Check sheet for the modelled part. Datum: model origin and axes. Units: mm. Face numbers are marked on the shaded views. Round coordinates to 2 decimals unless told otherwise and drop trailing zeros. Loops run counter-clockwise (first coordinate to the right, second up) from the corner with the lowest first, then second, coordinate; pieces in that order, holes last. Notation, with made-up numbers: (10, 39) - (43, 39) arc R12 cw to (43, 61) - close; hole circle Ø3 at (76, -39.75). An arc over 180 degrees is marked (long way). Put each result on its own line as item: value. Start each with the question number.
Item 1: Material ranges on line 1 along X through (y, z) = (1.15, 0); line 2 along X through (y, z) = (3.9, 0); line 3 along X through (y, z) = (4.8, -18), recorded low to high.
Item 2: Section check D-D, the plane z = -24.5. Record the cut outline in (x, y).
Item 3: Section check A-A, the plane y = 3.85. Record the cut outline in (x, z), and give its area (3 significant figures).
Item 4: Gauge pin test, flat ends, axial feed: pin 1 Ø0.9 at (x, z) = (-18, 18) entering from +Y; pin 2 Ø0.8 at (x, y) = (-1, 2) entering from +Z; pin 3 Ø4 at (x, z) = (33, 0) entering from -Y. Record the tip position at first contact, or that the pin passes through.
Item 5: Section check B-B, the plane z = 33.1. Record the cut outline in (x, y), and give its area (3 significant figures).
Item 6: Draft check along Z on the marked faces 1 and 2. Enter one of: pulls with the +Z half, pulls with the -Z half, needs draft (parallel to the pull), parting line crosses it, or undercut.
Item 7: Section check C-C, the plane x = -33.1. Record the cut outline in (y, z).
from build123d import *

# Parameters (mm, degrees)
SKETCH1_R           = 38.1
BOSS_EXTRUDE1_DEPTH = 5
SKETCH3_W           = 8.5
SKETCH3_H           = 20.2
CUT_EXTRUDE2_DEPTH  = 2.5
SKETCH4_W           = 5
SKETCH4_H           = 2
CUT_EXTRUDE4_DEPTH  = 54.939503149
SKETCH5_R           = 1.5
CUT_EXTRUDE5_DEPTH  = 3
SKETCH6_R           = 2.5
CUT_EXTRUDE6_DEPTH  = 3


with BuildPart() as part:
    # Sketch1 → Boss-Extrude1 (new body)
    with BuildSketch(Plane(origin=(0, 0, 0), x_dir=(1, 0, 0), z_dir=(0, 1, 0))):
        with Locations(Location((0, 0, 0), (0, 0, 270))):
            Circle(SKETCH1_R)
    extrude(amount=BOSS_EXTRUDE1_DEPTH)

    # Sketch3 → Cut-Extrude2 (cut)
    with BuildSketch(Plane(origin=(0, 5, 0), x_dir=(1, 0, 0), z_dir=(0, 1, 0))):
        with Locations((0, 7.5)):
            Rectangle(SKETCH3_W, SKETCH3_H)
    extrude(amount=-CUT_EXTRUDE2_DEPTH, mode=Mode.SUBTRACT)

    # Sketch4 → Cut-Extrude4 (cut, through all)
    with BuildSketch(Plane(origin=(0, 2.5, 0), x_dir=(1, 0, 0), z_dir=(0, 1, 0))):
        with Locations((0, -1.6)):
            Rectangle(SKETCH4_W, SKETCH4_H)
    extrude(amount=-CUT_EXTRUDE4_DEPTH, mode=Mode.SUBTRACT)

    # Sketch5 → Cut-Extrude5 (cut)
    with BuildSketch(Plane(origin=(0, 5, 0), x_dir=(1, 0, 0), z_dir=(0, 1, 0))):
        with Locations(Location((17.67766953, 17.67766953, 0), (0, 0, 270))):
            Circle(SKETCH5_R)
        with Locations(Location((-17.67766953, 17.67766953, 0), (0, 0, 270))):
            Circle(SKETCH5_R)
        with Locations(Location((-17.67766953, -17.67766953, 0), (0, 0, 270))):
            Circle(SKETCH5_R)
        with Locations(Location((17.67766953, -17.67766953, 0), (0, 0, 270))):
            Circle(SKETCH5_R)
    extrude(amount=-CUT_EXTRUDE5_DEPTH, mode=Mode.SUBTRACT)

    # Sketch6 → Cut-Extrude6 (cut)
    with BuildSketch(Plane.XZ):
        with Locations(Location((0, -33.1, 0), (0, 0, 270))):
            Circle(SKETCH6_R)
        with Locations(Location((33.1, 0, 0), (0, 0, 270))):
            Circle(SKETCH6_R)
        with Locations(Location((0, 33.1, 0), (0, 0, 270))):
            Circle(SKETCH6_R)
        with Locations(Location((-33.1, 0, 0), (0, 0, 270))):
            Circle(SKETCH6_R)
    extrude(amount=-CUT_EXTRUDE6_DEPTH, mode=Mode.SUBTRACT)


solid = part.part
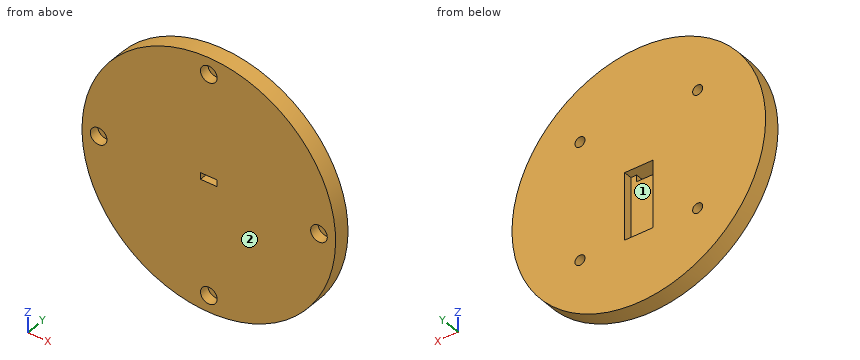
Check result:
1. line 1: -38.1 to -35.6, -30.6 to 30.6, 35.6 to 38.1
1. line 2: -38.1 to -4.25, 4.25 to 38.1
1. line 3: -33.58 to -19.14, -16.21 to 16.21, 19.14 to 33.58
2. outline: (-29.18, 0) - (29.18, 0) - (29.18, 5) - (-29.18, 5) - close
3. outline: circle Ø76.2 at (0, 0); hole circle Ø3 at (-17.68, -17.68); hole circle Ø3 at (-17.68, 17.68); hole (-4.25, -17.6) - (4.25, -17.6) - (4.25, 2.6) - (-4.25, 2.6) - close; hole circle Ø3 at (17.68, -17.68); hole circle Ø3 at (17.68, 17.68)
3. area: 4,360 mm²
4. pin 1: y = 2
4. pin 2: z = 38.1
4. pin 3: y = 3
5. outline: (-18.87, 0) - (-2.5, 0) - (-2.5, 3) - (2.5, 3) - (2.5, 0) - (18.87, 0) - (18.87, 5) - (-18.87, 5) - close
5. area: 174 mm²
6. face 1: undercut
6. face 2: needs draft
7. outline: (0, -18.87) - (5, -18.87) - (5, 18.87) - (0, 18.87) - (0, 2.5) - (3, 2.5) - (3, -2.5) - (0, -2.5) - close
